Part model, mm, in its own coordinate system. A direction names the side the tool comes from. Round coordinates to 2 decimals unless told otherwise and drop trailing zeros. Order: outer loops, then holes, each group sorted by start corner. A loop starts at its lowest first (then second) coordinate and runs counter-clockwise, first axis right, second up. Notation, with made-up numbers: M -4.75,56 L 1.25,56 A20 ccw 1.25,86 Z; hole C -3,56 d11. An arc over 180 degrees is marked long. Write each question's results on one line, items separated by ' | '. Start each with the question number.
1. Two-plate mould, pull along Z, no slides. Class faces 1 (the face through (25.348, -11.549, 0.089)), 2 (the face through (13, -2, 6.35)), 3 (the face through (12.5, 7.4, -13.8)): +Z half, -Z half, draft (parallel to the pull), parting line (faces both ways), or undercut.
2. Band-saw the part on C-C, the plane z = -26. List the corners of the cut face in (x, y), then the cut area to 3 significant figures.
3. Band-saw the part on A-A, the plane y = -12.7. List the corners of the cut face in (x, z) (3 decimals).
4. Drop flat-ended pins along their axis: pin 1 Ø3 at (y, z) = (-22.5, 1.5) entering from +X; pin 2 Ø4.5 at (y, z) = (-24, -0.5) entering from +X (3 decimals); pin 3 Ø2.5 at (x, y) = (10.5, 9.5) entering from -Z; pin 4 Ø1.5 at (x, y) = (17.5, -17.5) entering from +Z. Give the stop position or say it passes through.
5. Which spindle directions (+Z, -Z, +X, -X, +Y, -Y) get a long thin tool onto all of the face, cutting with end or side? Do faces 4 (the face through (20.617, -0.437, -0.089)), 5 (the face through (10, -3, -6.35)), 6 (the face through (19.955, -25.919, -0.089)), 7 (the face through (22.225, -24, 0)). Say none if no direction does.
6. Probe L1, parallel to X at y = -12.7, z = -0.75 (3 decimals); L2, parallel to Z at x = 13.75, y = -2.5; L3, parallel to Y at x = 3, z = 2. List the from-to ranges inside material, lowest first. Write a range as [from, to].
```python
from build123d import *

# Parameters (mm, degrees)
F0_W        = 6.35
F0_H        = 6.35
F0_H_2      = 31.75
F1_DEPTH    = 25.4
F3_DEPTH    = 12.7
F4_R        = 3.17499
F5_T1_DEPTH = 12.7
F6_R        = 6.35
F7_T1_DEPTH = 42.7131376889


# Not quite as in the source:
# - a fillet or chamfer that OpenCascade refuses, or shapes differently, is made with other operations: its cross-section is extruded or revolved along the edge and cut away or added
# - a fillet or chamfer is up to 0.001 mm smaller than in the source, because OpenCascade refuses the exact size


with BuildPart() as f1:
    # F0 (on Right) → F1 (new body)
    with BuildSketch(Plane.YZ):
        with Locations((3.175, 3.175)):
            Rectangle(F0_W, F0_H)
        with Locations((3.175, -15.875)):
            Rectangle(F0_W, F0_H_2)
        with BuildLine():
            Line((6.35, 6.35), (6.35, 0))
            Line((6.35, 0), (11.1125, 0))
            ThreePointArc((11.1125, 0), (7.1582593776, -15.6298064568), (7.4156091525, -31.75))
            Line((7.4156091525, -31.75), (10.4078971116, -31.75))
            ThreePointArc((10.4078971116, -31.75), (10.6800087855, -12.0972684736), (17.4625, 6.35))
            Line((17.4625, 6.35), (6.35, 6.35))
        make_face()
    extrude(amount=F1_DEPTH)

    # F2 (on face) → F3 (join)
    with BuildSketch(Plane.XY.offset(6.35)):
        with BuildLine():
            Line((19.05, 0), (6.35, 0))
            Line((6.35, 0), (6.35, -1.7014773719))
            ThreePointArc((6.35, -1.7014773719), (0.166760111, -10.6486838652), (3.175, -21.1002604126))
            ThreePointArc((3.175, -21.1002604126), (4.6568881715, -22.5284460682), (6.35, -23.6985226281))
            Line((6.35, -23.6985226281), (6.35, -19.7995158286))
            ThreePointArc((6.35, -19.7995158286), (12.7, -3.175), (19.05, -19.7995158286))
            Line((19.05, -19.7995158286), (19.05, -23.6985226281))
            ThreePointArc((19.05, -23.6985226281), (20.7431118285, -22.5284460682), (22.225, -21.1002604126))
            ThreePointArc((22.225, -21.1002604126), (25.233239889, -10.6486838652), (19.05, -1.7014773719))
            Line((19.05, -1.7014773719), (19.05, 0))
        make_face()
        with BuildLine():
            ThreePointArc((6.35, -23.6985226281), (4.6568881715, -22.5284460682), (3.175, -21.1002604126))
            Line((3.175, -21.1002604126), (3.175, -26.8735226281))
            Line((3.175, -26.8735226281), (6.35, -26.8735226281))
            Line((6.35, -26.8735226281), (6.35, -23.6985226281))
        make_face()
        with BuildLine():
            Line((22.225, -26.8735226281), (22.225, -21.1002604126))
            ThreePointArc((22.225, -21.1002604126), (20.7431118285, -22.5284460682), (19.05, -23.6985226281))
            Line((19.05, -23.6985226281), (19.05, -26.8735226281))
            Line((19.05, -26.8735226281), (22.225, -26.8735226281))
        make_face()
    extrude(amount=-F3_DEPTH)

    # F4 (radius 3.175 in the source; OpenCascade refuses exactly that, so slightly less here)
    f4_edges = [f1.edges().sort_by_distance(p)[0] for p in [
        (6.35, -26.873523, 0),
        (19.05, -26.873523, 0),
    ]]
    fillet(f4_edges, radius=F4_R)

    # F5: fillet of radius 3.175 on 4 edges, made by hand

    # F5_s2 → F5_t1 (join)
    with BuildSketch(Plane.XY.offset(-6.35)):
        with BuildLine():
            ThreePointArc((5.08, -2.54), (6.0148063314, -1.4199031657), (6.35, 0))
            Line((6.35, 0), (6.35, -1.7014773719))
            ThreePointArc((6.35, -1.7014773719), (5.7024286321, -2.1016984875), (5.08, -2.54))
        make_face()
        with BuildLine():
            ThreePointArc((20.32, -2.54), (19.3851936686, -1.4199031657), (19.05, 0))
            Line((19.05, 0), (19.05, -1.7014773719))
            ThreePointArc((19.05, -1.7014773719), (19.6975713679, -2.1016984875), (20.32, -2.54))
        make_face()
        with BuildLine():
            ThreePointArc((19.05, -3.175), (19.9799359697, -0.9299359697), (22.225, 0))
            Line((22.225, 0), (19.05, 0))
            Line((19.05, 0), (19.05, -3.175))
        make_face()
        with BuildLine():
            ThreePointArc((3.175, 0), (5.4200640303, -0.9299359697), (6.35, -3.175))
            Line((6.35, -3.175), (6.35, 0))
            Line((6.35, 0), (3.175, 0))
        make_face()
    extrude(amount=F5_T1_DEPTH)

    # F6
    f6_edges = [f1.edges().sort_by_distance(p)[0] for p in [
        (12.7, 17.4625, 6.35),
    ]]
    fillet(f6_edges, radius=F6_R)

    # F7: chamfer of 3.175 on 1 edges, made by hand

    # F7_s2 → F7_t1 (cut)
    with BuildSketch(Plane.YZ.offset(-8.6565688444)):
        with BuildLine():
            Line((10.772273237, -31.8355341736), (6.9175477916, -28.3233800406))
            Line((6.9175477916, -28.3233800406), (6.8543218231, -28.3292729944))
            ThreePointArc((6.8543218231, -28.3292729944), (7.1217830499, -30.0420734544), (7.3528018544, -31.759353786))
            Line((7.3528018544, -31.759353786), (7.4156091525, -31.8135))
            ThreePointArc((7.4156091525, -31.8135), (9.0939411948, -31.8135), (10.772273237, -31.8990341736))
            Line((10.772273237, -31.8990341736), (10.772273237, -31.8355341736))
        make_face()
    extrude(amount=F7_T1_DEPTH, mode=Mode.SUBTRACT)


solid = f1.part
```
Solution:
1) face 1: draft | face 2: +Z half | face 3: undercut
2) outline: M 0,0 L 25.4,0 L 25.4,6.35 L 0,6.35 Z; M 0,6.83 L 25.4,6.83 L 25.4,9.8 L 0,9.8 Z | area: 237 mm^2
3) outline: M 0,-6.35 L 3.175,-6.35 L 3.175,6.35 L 0,6.35 Z; M 22.225,-6.35 L 25.4,-6.35 L 25.4,6.35 L 22.225,6.35 Z
4) pin 1: x = 22.31 | pin 2: x = 22.225 | pin 3: z = -31.46 | pin 4: through
5) face 4: +Z, -Z, +X | face 5: -Z, +X, -X, -Y | face 6: +Z, -Z, -Y | face 7: +Z, -Z, +X, -Y
6) L1: [0, 3.175], [22.225, 25.4] | L2: [-6.35, 6.35] | L3: [-20.9, -4.5], [0, 13.5]
